The model under review builds one solid part; all positions refer to its coordinate system, in mm. A direction names the side the tool comes from. Coordinates: 2 decimals unless noted, no trailing zeros. Write each loop counter-clockwise with the first axis right and the second up, starting at its lowest first coordinate (ties: lowest second). Pieces come first, ordered by that corner, then holes. Notation, with made-up numbers: M 33.25,-0.75 L 54.25,-0.75 A37 cw 54.25,38.25 Z; hole C -30,-13.5 d5. An arc over 180 degrees is marked long. Answer as a JSON object with one key per item and string values.
```python
from build123d import *

# Parameters (mm, degrees)
BOSS_EXTRUDE1_DEPTH = 1.5
SKETCH10_R          = 4.9
BOSS_EXTRUDE2_DEPTH = 5


with BuildPart() as part:
    # Sketch1 → Boss-Extrude1 (new body)
    with BuildSketch(Plane.XY):
        Polygon((0, 6), (0.314446676, 0), (1.497941481, 0), (1.657221927, 3.039251967), (2.042586863, 3.65596478), (2.769801294, 3.65596478), (3.155166229, 3.039251967), (3.314446676, 0), (4.497941481, 0), (4.657221927, 3.039251967), (5.042586863, 3.65596478), (5.769801294, 3.65596478), (6.155166229, 3.039251967), (6.314446676, 0), (7.497941481, 0), (7.657221927, 3.039251967), (8.042586863, 3.65596478), (8.769801294, 3.65596478), (9.155166229, 3.039251967), (9.314446676, 0), (10.497941481, 0), (10.657221927, 3.039251967), (11.042586863, 3.65596478), (11.769801294, 3.65596478), (12.155166229, 3.039251967), (12.314446676, 0), (13.497941481, 0), (13.657221927, 3.039251967), (14.042586863, 3.65596478), (16.269801294, 3.65596478), (16.655166229, 3.039251967), (16.814446676, 0), (17.997941481, 0), (18.312388157, 6), (18.312388157, 17.6), (0, 17.6), align=None)
    extrude(amount=BOSS_EXTRUDE1_DEPTH)

    # Sketch10 → Boss-Extrude2 (add)
    with BuildSketch(Plane.XY):
        with Locations((9.112388157, 12)):
            Circle(SKETCH10_R)
    extrude(amount=-BOSS_EXTRUDE2_DEPTH)


solid = part.part
```
(1) For faces 4 (the face through (8.05, 7.217, -2.465)), 5 (the face through (9, 12, -5)), 6 (the face through (9.234, 1.541, 0.74)), list the 3-axis set-ups (+Z, -Z, +X, -X, +Y, -Y) from which the entire face can be reached by the end or side of a thin tool; tool diameter is ignored.
Results list:
{"face 4": "-Z", "face 5": "-Z, +X, -X, +Y, -Y", "face 6": "+Z, -Z, -Y"}
(2) Add section C-C on z = -3.25. Give the boundary of the cut face in (x, y).
Results list:
{"outline": "C 9.11,12 d9.8"}
(3) Add section D-D on y = 16. Give the boundary of the cut face in (x, z).
Results list:
{"outline": "M 0,0 L 6.28,0 L 6.28,-5 L 11.94,-5 L 11.94,0 L 18.31,0 L 18.31,1.5 L 0,1.5 Z"}
(4) For pin 1 Ø1.5 at (x, y) = (14.5, 3.5) entering from -Z; pin 2 Ø0.8 at (x, z) = (5.5, 0.5) entering from -Y; pin 3 Ø0.8 at (x, z) = (15.5, 0.5) entering from -Y; pin 4 Ø2 at (y, z) = (6, -3.5) entering from -X, all flat-tipped, find the tip position at first contact; note any pin that passes through.
Results list:
{"pin 1": "z = 0", "pin 2": "y = 3.45", "pin 3": "y = 3.66", "pin 4": "through"}
(5) Add section A-A on y = 12. Give the boundary of the cut face in (x, z).
Results list:
{"outline": "M 0,0 L 4.21,0 L 4.21,-5 L 14.01,-5 L 14.01,0 L 18.31,0 L 18.31,1.5 L 0,1.5 Z"}
(6) Wall thickness on line 1 along X through (y, z) = (3.25, 1.25); line 2 along Z through (x, y) = (3, 6); line 3 along X through (y, z) = (1.25, 1): over which ranges is each line inside the solid? List them lowest first. Write a range as from..to.
Results list:
{"line 1": "0.14..1.79, 3.02..4.79, 6.02..7.79, 9.02..10.79, 12.02..13.79, 16.52..18.17", "line 2": "0..1.5", "line 3": "0.25..1.56, 3.25..4.56, 6.25..7.56, 9.25..10.56, 12.25..13.56, 16.75..18.06"}
(7) Draft analysis for pull direction X (two halves, no side actions). For faces 1 (the face through (12.234, 1.541, 0.74)), 2 (the face through (7, 7, 0)), 3 (the face through (0.155, 3.042, 0.74)), state which applies: released by +X, released by -X, zero draft, split by the parting line, or undercut.
Results list:
{"face 1": "undercut", "face 2": "zero draft", "face 3": "released by -X"}
(8) Add section B-B on x = 17.25. Give the boundary of the cut face in (y, z).
Results list:
{"outline": "M 0,0 L 17.6,0 L 17.6,1.5 L 0,1.5 Z"}
